Geometry check sheet. Reference: the model listing, model coordinates, mm. Round coordinates to 2 decimals unless told otherwise and drop trailing zeros. Order: outer loops, then holes, each group sorted by start corner. A loop starts at its lowest first (then second) coordinate and runs counter-clockwise, first axis right, second up. Notation, with made-up numbers: (60.5, 2) -> (117.5, 2) arc R28 ccw to (117.5, 24) -> close; hole circle Ø1 at (29.5, -23.75). An arc over 180 degrees is marked (long way). Use a Markdown table: item, result. Add a question column.
Item 1: Sectioned sample at C-C, the plane z = 1.4. Record the cut outline in (x, y) (3 decimals).
Item 2: Sectioned sample at B-B, the plane y = 39. Record the cut outline in (x, z), and give its area (3 significant figures).
Item 3: Sectioned sample at D-D, the plane x = 7. Record the cut outline in (y, z).
Item 4: Gauge pin test, flat ends, axial feed: pin 1 Ø12 at (x, y) = (48.5, 17.5) entering from +Z; pin 2 Ø10 at (x, y) = (8, 80.5) entering from +Z; pin 3 Ø1 at (x, y) = (70, 84.5) entering from +Z. Record the tip position at first contact, or that the pin passes through.
Item 5: Sectioned sample at A-A, the plane x = 18.5. Record the cut outline in (y, z).
Item 6: Material ranges on probe 1 along Y at (x, z) = (46, 0.3); probe 2 along X at (y, z) = (100.5, 0.7) (3 decimals); probe 3 along Y at (x, z) = (75.5, 0.4) (3 decimals), recorded low to high. Write a range as [from, to].
Item 7: Mould release check, pull along Y, two halves, no side actions. Record for faces 1 (the flat face through (73, 52, 0)), 2 (the flat face through (8.6, 55.2, 0.5)): pulls with the +Y half, pulls with the -Y half, needs draft (parallel to the pull), parting line crosses it, or undercut.
from build123d import *

# Parameters (mm, degrees)
F0_W     = 68
F0_H     = 93
F0_W_2   = 60
F0_H_2   = 85
F1_DEPTH = 0.5
F0_W_3   = 78
F0_H_3   = 103
F0_R     = 1.125
F0_R_2   = 0.875
F2_DEPTH = 1
F3_DEPTH = 1.8


with BuildPart() as f1:
    # F0 (on Top) → F1 (new body)
    with BuildSketch(Plane.XY):
        with Locations((39, 51.5)):
            Rectangle(F0_W, F0_H)
        with Locations((39, 51.5)):
            Rectangle(F0_W_2, F0_H_2, mode=Mode.SUBTRACT)
    extrude(amount=F1_DEPTH)

    # F0 (on Top) → F2 (join)
    with BuildSketch(Plane.XY):
        with Locations((39, 51.5)):
            Rectangle(F0_W_3, F0_H_3)
        with Locations((2.5, 2.5)):
            Circle(F0_R, mode=Mode.SUBTRACT)
        with Locations((75.5, 2.5)):
            Circle(F0_R_2, mode=Mode.SUBTRACT)
        with Locations((39, 51.5)):
            Rectangle(F0_W, F0_H, mode=Mode.SUBTRACT)
        with Locations((2.5, 100.5)):
            Circle(F0_R_2, mode=Mode.SUBTRACT)
        with Locations((75.5, 100.5)):
            Circle(F0_R, mode=Mode.SUBTRACT)
    extrude(amount=F2_DEPTH)

    # F0 (on Top) → F3 (join)
    with BuildSketch(Plane.XY):
        with Locations((75.5, 2.5)):
            Circle(F0_R_2)
        with Locations((2.5, 100.5)):
            Circle(F0_R_2)
    extrude(amount=F3_DEPTH)


solid = f1.part
Found:
| question | item | result |
|---|---|---|
| 1 | outline | circle Ø1.75 at (2.5, 100.5); circle Ø1.75 at (75.5, 2.5) |
| 2 | outline | (0, 0) -> (9, 0) -> (9, 0.5) -> (5, 0.5) -> (5, 1) -> (0, 1) -> close; (69, 0) -> (78, 0) -> (78, 1) -> (73, 1) -> (73, 0.5) -> (69, 0.5) -> close |
| 2 | area | 14.0 mm2 |
| 3 | outline | (0, 0) -> (103, 0) -> (103, 1) -> (98, 1) -> (98, 0.5) -> (5, 0.5) -> (5, 1) -> (0, 1) -> close |
| 4 | pin 1 | passes through |
| 4 | pin 2 | stops at z = 1 |
| 4 | pin 3 | stops at z = 0.5 |
| 5 | outline | (0, 0) -> (9, 0) -> (9, 0.5) -> (5, 0.5) -> (5, 1) -> (0, 1) -> close; (94, 0) -> (103, 0) -> (103, 1) -> (98, 1) -> (98, 0.5) -> (94, 0.5) -> close |
| 6 | probe 1 | y = [0, 9], [94, 103] |
| 6 | probe 2 | x = [0, 74.375], [76.625, 78] |
| 6 | probe 3 | y = [0, 99.375], [101.625, 103] |
| 7 | face 1 | needs draft |
| 7 | face 2 | undercut |
